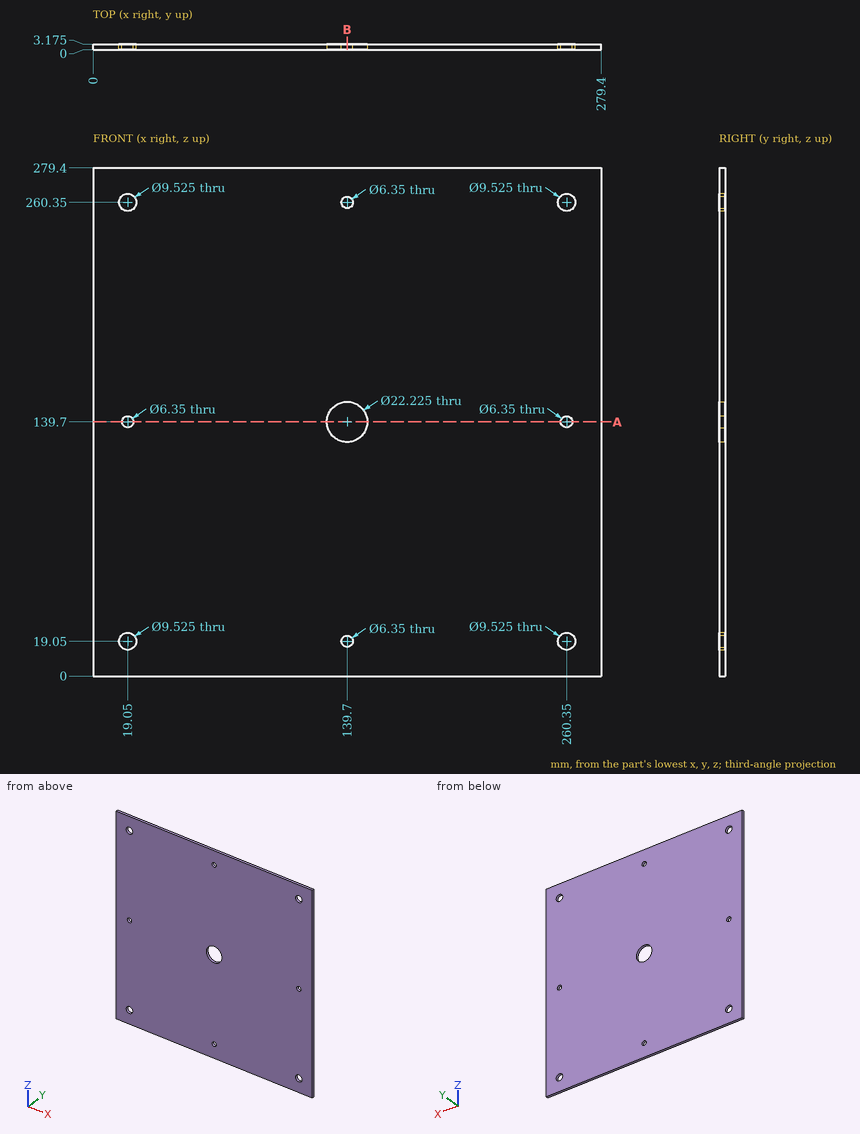
Verification items for this drawing (mm, ordinates from the low corner). Give positions to 0.01 mm unless a question says otherwise; leave off trailing zeros. Write each loop counter-clockwise with the first axis right and the second up, starting at its lowest first coordinate (ties: lowest second). Pieces come first, ordered by that corner, then holes. Notation, with made-up numbers: (-37.75, 28.5) -> (-14.75, 28.5) arc R16 ccw to (-14.75, 35.5) -> close; hole circle Ø6 at (84.25, 7). An arc over 180 degrees is marked (long way). Use one line per item in the form item = value.
Item 1: Scan lines: line 1 (Z direction, x = 19.05, y = 0.8) (1 decimal); line 2 (X direction, y = 2.75, z = 17). Record each from-to range of solid material in increasing order.
Results list:
line_1 = 0 to 14.3, 23.8 to 136.5, 142.9 to 255.6, 265.1 to 279.4
line_2 = 0 to 14.75, 23.35 to 137.28, 142.12 to 256.05, 264.65 to 279.4
Item 2: Depth check by flat-ended pin: pin 1 Ø4 at (x, z) = (195, 225) entering from -Y; pin 2 Ø7.5 at (x, z) = (19.05, 19.05) entering from -Y. Enter the tip coordinate at first touch or a pass-through.
Results list:
pin_1 = 0
pin_2 = through
Item 3: Sectioned sample at A-A on z = 139.7. Enter the section's corners in (x, y) (1 decimal), plus the area to 3 significant figures.
Results list:
outline = (0, 0) -> (15.9, 0) -> (15.9, 3.2) -> (0, 3.2) -> close; (22.2, 0) -> (128.6, 0) -> (128.6, 3.2) -> (22.2, 3.2) -> close; (150.8, 0) -> (257.2, 0) -> (257.2, 3.2) -> (150.8, 3.2) -> close; (263.5, 0) -> (279.4, 0) -> (279.4, 3.2) -> (263.5, 3.2) -> close
area = 776 mm2
Item 4: Sectioned sample at B-B on x = 139.7. Enter the section's corners in (y, z) (1 decimal), plus the area to 3 significant figures.
Results list:
outline = (0, 0) -> (3.2, 0) -> (3.2, 15.9) -> (0, 15.9) -> close; (0, 22.2) -> (3.2, 22.2) -> (3.2, 128.6) -> (0, 128.6) -> close; (0, 150.8) -> (3.2, 150.8) -> (3.2, 257.2) -> (0, 257.2) -> close; (0, 263.5) -> (3.2, 263.5) -> (3.2, 279.4) -> (0, 279.4) -> close
area = 776 mm2
